Geometry: see drawing. Coordinates: mm, zero at the bounding-box minimum. Coordinates: 2 decimals unless noted, no trailing zeros. Loops run counter-clockwise (first coordinate to the right, second up) from the corner with the lowest first, then second, coordinate; pieces in that order, holes last.
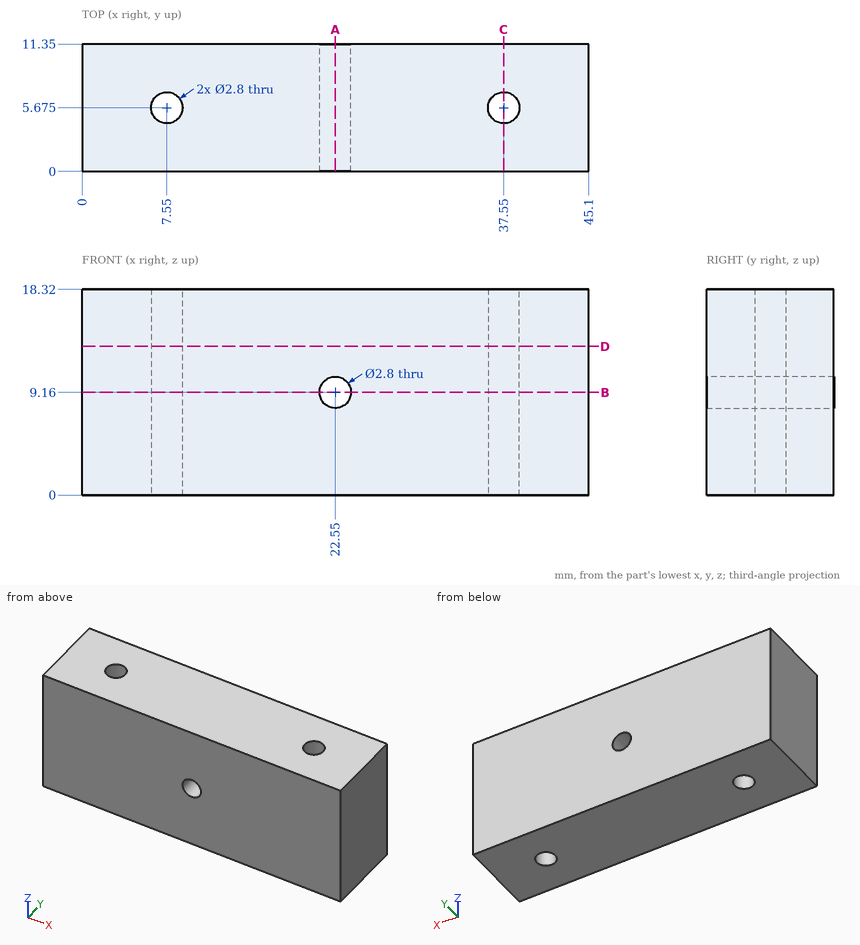
Item 1: Section query C-C (x = 37.55). Output: boundary loops of the cut face in (y, z) (3 decimals).
Result:
outline: (0, 0) - (4.275, 0) - (4.275, 18.32) - (0, 18.32) - close; (7.075, 0) - (11.35, 0) - (11.35, 18.32) - (7.075, 18.32) - close
Item 2: Section query B-B (z = 9.16). Output: boundary loops of the cut face in (x, y) (3 decimals), then the cut area to 3 significant figures.
Result:
outline: (0, 0) - (21.15, 0) - (21.15, 11.35) - (0, 11.35) - close; (23.95, 0) - (45.1, 0) - (45.1, 11.35) - (23.95, 11.35) - close; hole circle Ø2.8 at (7.55, 5.675); hole circle Ø2.8 at (37.55, 5.675)
area: 468 mm2
Item 3: Line query: L1, parallel to Y at x = 37.55, z = 9.75 (3 decimals); L2, parallel to X at y = 4.5, z = 14; L3, parallel to X at y = 4.75, z = 8.75. Output: solid intervals per line, ascending.
Result:
L1: y = 0 to 4.275, 7.075 to 11.35
L2: x = 0 to 6.79, 8.31 to 36.79, 38.31 to 45.1
L3: x = 0 to 6.5, 8.6 to 21.21, 23.89 to 36.5, 38.6 to 45.1
Item 4: Section query D-D (z = 13.25). Output: boundary loops of the cut face in (x, y) (3 decimals).
Result:
outline: (0, 0) - (45.1, 0) - (45.1, 11.35) - (0, 11.35) - close; hole circle Ø2.8 at (7.55, 5.675); hole circle Ø2.8 at (37.55, 5.675)
Item 5: Section query A-A (x = 22.55). Output: boundary loops of the cut face in (y, z).
Result:
outline: (0, 0) - (11.35, 0) - (11.35, 7.76) - (0, 7.76) - close; (0, 10.56) - (11.35, 10.56) - (11.35, 18.32) - (0, 18.32) - close
